The model under review builds one solid part; all positions refer to its coordinate system, in mm. Coordinates: 2 decimals unless noted, no trailing zeros. Order: outer loops, then holes, each group sorted by start corner. A loop starts at its lowest first (then second) coordinate and runs counter-clockwise, first axis right, second up.
Autodesk Inventor part; units mm, degrees
ref_plane "YZ Plane" through (0, 0, 0) normal (1, 0, 0) x (0, 1, 0)
ref_plane "XZ Plane" through (0, 0, 0) normal (0, 1, 0) x (-1, 0, 0)
ref_plane "XY Plane" through (0, 0, 0) normal (0, 0, 1) x (1, 0, 0)
sketch "Sketch1" plane through (0, 0, 0) normal (0, 1, 0) x (-1, 0, 0)
  circle A0 centre (0, 0) radius 101.6
  circle A1 centre (0, 0) radius 95.25
  dimension "d0" = 203.2
  dimension "d1" = 190.5
extrude "Extrusion1" add sketch "Sketch1" along normal blind 7.62
sketch "Sketch2" plane through (0, 7.62, 0) normal (0, 1, 0) x (1, 0, 0)
  line L0 (0, 0) -> (69.597, 69.597) construction
  line L1 (0, 0) -> (98.425, 0) construction
  point P0 (71.1594, 93.9158)
  dimension "d4" = 98.425
  dimension "d5" = 45
hole "Hole1" at (69.597, 7.62, -69.597) at (71.1594, 7.62, -93.9158) direction (0, -1, 0) diameter 2.2606 end through all
pattern_circular "Circular Pattern1" count 6 over 360 about axis through (0, 0, 0) along (0, 1, 0) of "Hole1"
properties part number "4K sheild rim" material "Brass, Soft Yellow"
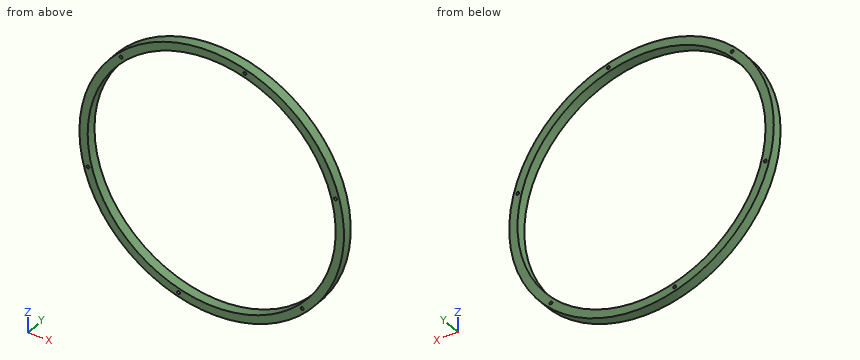
(1) We need section A-A, the plane z = 0. Write out the cut boundary in (x, y), and give its area (3 significant figures).
A:
outline: (-101.6, 0) - (-95.25, 0) - (-95.25, 7.62) - (-101.6, 7.62) - close; (95.25, 0) - (101.6, 0) - (101.6, 7.62) - (95.25, 7.62) - close
area: 96.8 mm2
(2) We need section B-B, the plane x = 0. Write out the cut boundary in (y, z), and give its area (3 significant figures).
A:
outline: (0, -101.6) - (7.62, -101.6) - (7.62, -95.25) - (0, -95.25) - close; (0, 95.25) - (7.62, 95.25) - (7.62, 101.6) - (0, 101.6) - close
area: 96.8 mm2
(3) For pin 1 Ø2 at (x, y) = (-65, 6) entering from -Z; pin 2 Ø1.4 at (x, z) = (25.47, 95.07) entering from -Y; pin 3 Ø4 at (x, y) = (50, 3) entering from -Z; pin 4 Ø1 at (x, y) = (-6, 5) entering from -Z, all flat-tipped, find the tip position at first contact; note any pin that passes through.
A:
pin 1: stops at z = -78.91
pin 2: passes through
pin 3: stops at z = -89.55
pin 4: stops at z = -101.45
(4) We need section C-C, the plane y = 5.75. Write out the cut boundary in (x, z).
A:
outline: circle Ø203.2 at (0, 0); hole circle Ø2.26 at (-95.07, -25.47); hole circle Ø190.5 at (0, 0); hole circle Ø2.26 at (-69.6, 69.6); hole circle Ø2.26 at (-25.47, -95.07); hole circle Ø2.26 at (25.47, 95.07); hole circle Ø2.26 at (69.6, -69.6); hole circle Ø2.26 at (95.07, 25.47)
(5) Wall thickness on probe 1 along Z at (x, y) = (-25, 2); probe 2 along Z at (x, y) = (1, 3.5); probe 3 along X at (y, z) = (3, -38): over which ranges is each line inside the solid? List them lowest first.
A:
probe 1: z = -98.48 to -96.1, -94.05 to -91.91, 91.91 to 98.48
probe 2: z = -101.6 to -95.24, 95.24 to 101.6
probe 3: x = -94.23 to -87.34, 87.34 to 94.23
